Input: dimensioned drawing with shaded views. Units: mm. Origin: part minimum x, y, z. Give positions to 0.01 mm unless a question says otherwise; leave off trailing zeros. Write each loop counter-clockwise with the first axis right and the second up, starting at its lowest first coordinate (ties: lowest second). Pieces come first, ordered by that corner, then holes. Notation, with made-up numbers: (60, 12) -> (104, 12) arc R12 ccw to (104, 23) -> close; hole circle Ø7 at (-22, -19). An arc over 180 degrees is marked (long way). Answer in a Markdown table with one row per item. Add a question column.
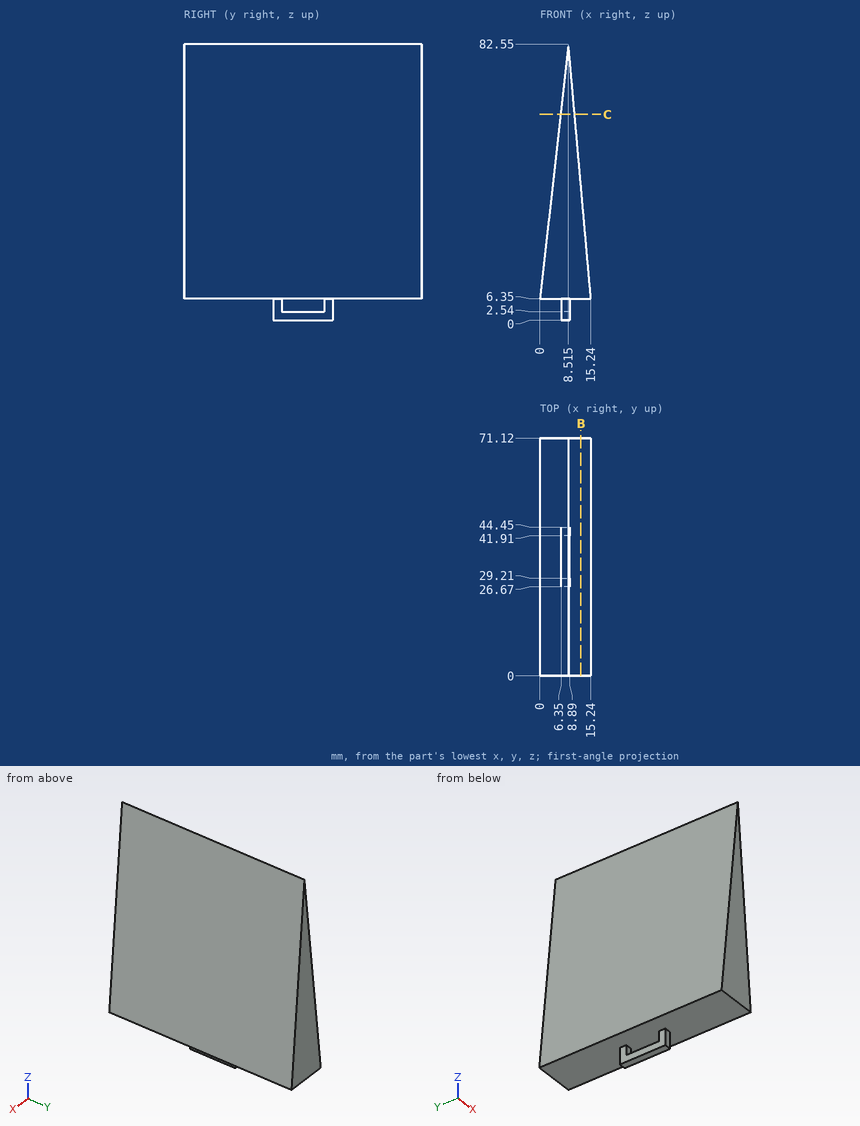
Q1. Contact query for flat-ended pins moving along their axis: pin 1 Ø2 at (x, z) = (7.5, 4.5) entering from -Y; pin 2 Ø5 at (y, z) = (50.5, 13) entering from -X; pin 3 Ø1.9 at (y, z) = (39, 2.5) entering from -X; pin 4 Ø3 at (x, z) = (3, 49) entering from -Y. Output: stop coordinate, or through.
Q2. Section B-B on x = 12.25. Return loops of the section in (y, z).
Q3. Line query: probe 1 along Y at (x, z) = (8.75, 5); probe 2 along X at (y, z) = (65.5, 58); probe 3 along X at (y, z) = (10.5, 78.5). Output: solid intervals per line, ascending. Write a range as from..to.
Q4. Section C-C on z = 61.5. Return loops of the section in (x, y).
Checks:
| question | item | result |
|---|---|---|
| 1 | pin 1 | y = 26.67 |
| 1 | pin 2 | x = 0.46 |
| 1 | pin 3 | x = 6.35 |
| 1 | pin 4 | through |
| 2 | outline | (0, 6.35) -> (71.12, 6.35) -> (71.12, 40.23) -> (0, 40.23) -> close |
| 3 | probe 1 | 26.67..29.21, 41.91..44.45 |
| 3 | probe 2 | 5.77..10.68 |
| 3 | probe 3 | 8.06..8.87 |
| 4 | outline | (6.16, 0) -> (10.37, 0) -> (10.37, 71.12) -> (6.16, 71.12) -> close |
